Read the model definition and answer for the solid it produces. Units are mm, in the model's axes. A direction names the side the tool comes from. Round coordinates to 2 decimals unless told otherwise and drop trailing zeros. Write each loop counter-clockwise with the first axis right and the second up, starting at its lowest first coordinate (ties: lowest second). Pieces come first, ordered by that corner, then holes. Notation, with made-up numbers: (-6, -26.75) - (35, -26.75) arc R23 ccw to (35, 1.25) - close; hole circle Ø2 at (43.5, 45). An arc over 180 degrees is marked (long way). Answer as CSV lines item,"result". Start each with the question number.
1) Which of the six approach directions +Z, -Z, +X, -X, +Y, -Y give full straight-line access (tool end or side, diameter ignored) to faces 4 (the flat face through (-2.3, -2.9, -0.1)), 5 (the flat face through (-5, 7.5, 0))?
2) Consider line 1 along Y through (x, z) = (5.5, 3.5); line 2 along Y through (x, z) = (7.25, -6.5); line 3 along Y through (x, z) = (-3.75, 0.25). Determine where each line is inside the solid, lowest interval first.
3) Find section C-C on y = -5.5. Determine the outline of the cut face in (x, z).
4) Each of these flat-tipped pins is pushed along its axis until it touches: pin 1 (1.7 mm diameter, centred on x = 0, z = 3, fed in from +Y); pin 2 (6 mm diameter, centred on x = 4.5, y = -2.5, fed in from -Z). Where does it stop, or does it pass through?
5) For a pull along X with two mould halves and no side action, classify faces 1 (the flat face through (5, 2.9, 0)), 2 (the flat face through (5, -7.5, 0)), 3 (the flat face through (-7.5, 5, 0)) as +X half, -X half, draft (parallel to the pull), parting line (faces both ways), or undercut.
6) Find section B-B on y = 0. Determine the outline of the cut face in (x, z), then the cut area to 3 significant figures.
7) Find section A-A on x = -0.75. Determine the outline of the cut face in (y, z), then the cut area to 3 significant figures.
Autodesk Fusion 360 part; units mm, degrees
sketch "Cross Section" plane through (0, 0, 0) normal (0, 0, 1) x (1, 0, 0)
  line L0 (-7.5, -7.5) -> (7.5, -7.5)
  line L1 (7.5, -7.5) -> (7.5, 7.5)
  line L2 (7.5, 7.5) -> (-7.5, 7.5)
  line L3 (-7.5, -1.8) -> (-7.5, -7.5)
  line L4 (-7.5, -7.5) -> (7.5, 7.5) construction
  line L5 (7.5, -7.5) -> (-7.5, 7.5) construction
  line L6 (-7.2, 1.5) -> (-6.8, 1.5)
  line L7 (-6.5, 1.8) -> (-6.5, 2.9)
  line L8 (-6.5, 2.9) -> (-3.5, 2.9)
  line L9 (-3.5, 2.9) -> (-2.3, 1.7)
  line L10 (-2.3, 1.7) -> (-2.3, -1.7)
  line L11 (-2.3, -1.7) -> (-3.5, -2.9)
  line L12 (-3.5, -2.9) -> (-6.5, -2.9)
  line L13 (-6.5, -2.9) -> (-6.5, -1.8)
  line L14 (-6.8, -1.5) -> (-7.2, -1.5)
  line L15 (-2.3, 0) -> (-7.5, 0) construction
  circle A0 centre (0, 0) radius 1.25
  circle A1 centre (-5.5, 5.5) radius 1.5
  line L16 (-7.5, -7.5) -> (-7.5, -1.5)
  line L17 (-7.5, 1.8) -> (-7.5, 7.5)
  arc A2 (-7.5, 1.8) -> (-7.2, 1.5) centre (-7.2, 1.8) ccw
  arc A3 (-6.8, 1.5) -> (-6.5, 1.8) centre (-6.8, 1.8) ccw
  arc A4 (-6.5, -1.8) -> (-6.8, -1.5) centre (-6.8, -1.8) ccw
  arc A5 (-7.2, -1.5) -> (-7.5, -1.8) centre (-7.2, -1.8) ccw
  arc A6 (-1.8, -7.5) -> (-1.5, -7.2) centre (-1.8, -7.2) ccw
  line L18 (-1.5, -7.2) -> (-1.5, -6.8)
  line L19 (2.9, -6.5) -> (1.8, -6.5)
  arc A7 (1.8, -6.5) -> (1.5, -6.8) centre (1.8, -6.8) ccw
  line L20 (1.5, -6.8) -> (1.5, -7.2)
  arc A8 (1.5, -7.2) -> (1.8, -7.5) centre (1.8, -7.2) ccw
  line L21 (2.9, -3.5) -> (2.9, -6.5)
  line L22 (1.7, -2.3) -> (2.9, -3.5)
  line L23 (-1.7, -2.3) -> (1.7, -2.3)
  line L24 (-2.9, -3.5) -> (-1.7, -2.3)
  line L25 (-2.9, -6.5) -> (-2.9, -3.5)
  line L26 (-1.8, -6.5) -> (-2.9, -6.5)
  arc A9 (-1.5, -6.8) -> (-1.8, -6.5) centre (-1.8, -6.8) ccw
  line L27 (7.5, -7.5) -> (1.5, -7.5)
  line L28 (-1.8, -7.5) -> (-7.5, -7.5)
  circle A10 centre (-5.5, -5.5) radius 1.5
  arc A11 (7.5, -1.8) -> (7.2, -1.5) centre (7.2, -1.8) ccw
  line L29 (7.2, -1.5) -> (6.8, -1.5)
  line L30 (6.5, 2.9) -> (6.5, 1.8)
  arc A12 (6.5, 1.8) -> (6.8, 1.5) centre (6.8, 1.8) ccw
  line L31 (6.8, 1.5) -> (7.2, 1.5)
  arc A13 (7.2, 1.5) -> (7.5, 1.8) centre (7.2, 1.8) ccw
  line L32 (3.5, 2.9) -> (6.5, 2.9)
  line L33 (2.3, 1.7) -> (3.5, 2.9)
  line L34 (2.3, -1.7) -> (2.3, 1.7)
  line L35 (3.5, -2.9) -> (2.3, -1.7)
  line L36 (6.5, -2.9) -> (3.5, -2.9)
  line L37 (6.5, -1.8) -> (6.5, -2.9)
  arc A14 (6.8, -1.5) -> (6.5, -1.8) centre (6.8, -1.8) ccw
  line L38 (7.5, 7.5) -> (7.5, 1.5)
  line L39 (7.5, -1.8) -> (7.5, -7.5)
  circle A15 centre (5.5, -5.5) radius 1.5
  arc A16 (1.8, 7.5) -> (1.5, 7.2) centre (1.8, 7.2) ccw
  line L40 (1.5, 7.2) -> (1.5, 6.8)
  line L41 (-2.9, 6.5) -> (-1.8, 6.5)
  arc A17 (-1.8, 6.5) -> (-1.5, 6.8) centre (-1.8, 6.8) ccw
  line L42 (-1.5, 6.8) -> (-1.5, 7.2)
  arc A18 (-1.5, 7.2) -> (-1.8, 7.5) centre (-1.8, 7.2) ccw
  line L43 (-2.9, 3.5) -> (-2.9, 6.5)
  line L44 (-1.7, 2.3) -> (-2.9, 3.5)
  line L45 (1.7, 2.3) -> (-1.7, 2.3)
  line L46 (2.9, 3.5) -> (1.7, 2.3)
  line L47 (2.9, 6.5) -> (2.9, 3.5)
  line L48 (1.8, 6.5) -> (2.9, 6.5)
  arc A19 (1.5, 6.8) -> (1.8, 6.5) centre (1.8, 6.8) ccw
  line L49 (-7.5, 7.5) -> (-1.5, 7.5)
  line L50 (1.8, 7.5) -> (7.5, 7.5)
  circle A20 centre (5.5, 5.5) radius 1.5
  dimension "d2" = 3
  dimension "d3" = 5.2
  dimension "d4" = 5.8
  dimension "d5" = 7.5
  dimension "d6" = 1
  dimension "d7" = 135
  dimension "d8" = 3
  dimension "d9" = 7.5
  dimension "d10" = 2.5
  dimension "d11" = 3
  dimension "d12" = 2
  dimension "d47" = 15
  dimension "d50" = 0.3
  dimension "d52" = 360
extrude "Extrude1" add sketch "Cross Section" along normal mid plane 15 contours L0 L1 L2 L3 L6 L7 L8 L9 L10 L11 L12 L13 L14 L16 L17 A2 A3 A4 A5 A6 L18 L19 A7 L20 A8 L21 L22 L23 L24 L25 L26 A9 L27 L28 A11 L29 L30 A12 L31 A13 L32 L33 L34 L35 L36 L37 A14 L38 L39 A16 L40 L41 A17 L42 A18 L43 L44 L45 L46 L47 L48 A19 L49 L50
equation "Extrusion_Length = 15 mm"
equation "d20 = Extrusion_Length"
Check values:
1,face 4,"+Z, -Z"
1,face 5,"+Z, -Z, +X, -X, +Y"
2,line 1,"y = -7.5 to -7, -4 to -2.9, 2.9 to 4, 7 to 7.5"
2,line 2,"y = -7.5 to -1.5, 1.5 to 7.5"
2,line 3,"y = -7.5 to -2.9, 2.9 to 7.5"
3,outline,"(-7.5, -7.5) - (-7, -7.5) - (-7, 7.5) - (-7.5, 7.5) - close; (-4, -7.5) - (-2.9, -7.5) - (-2.9, 7.5) - (-4, 7.5) - close; (2.9, -7.5) - (4, -7.5) - (4, 7.5) - (2.9, 7.5) - close; (7, -7.5) - (7.5, -7.5) - (7.5, 7.5) - (7, 7.5) - close"
4,pin 1,"stops at y = 2.3"
4,pin 2,"stops at z = -7.5"
5,face 1,"undercut"
5,face 2,"draft"
5,face 3,"-X half"
6,outline,"(-2.3, -7.5) - (-1.25, -7.5) - (-1.25, 7.5) - (-2.3, 7.5) - close; (1.25, -7.5) - (2.3, -7.5) - (2.3, 7.5) - (1.25, 7.5) - close"
6,area,"31.5 mm^2"
7,outline,"(-2.3, -7.5) - (-1, -7.5) - (-1, 7.5) - (-2.3, 7.5) - close; (1, -7.5) - (2.3, -7.5) - (2.3, 7.5) - (1, 7.5) - close"
7,area,"39.0 mm^2"
